Could you check a few things on this drawing? It's one solid part, dimensions in mm from its lowest x, y, z. Coordinates: 2 decimals unless noted, no trailing zeros. Write each loop counter-clockwise with the first axis right and the second up, starting at its lowest first coordinate (ties: lowest second). Pieces come first, ordered by that corner, then holes.
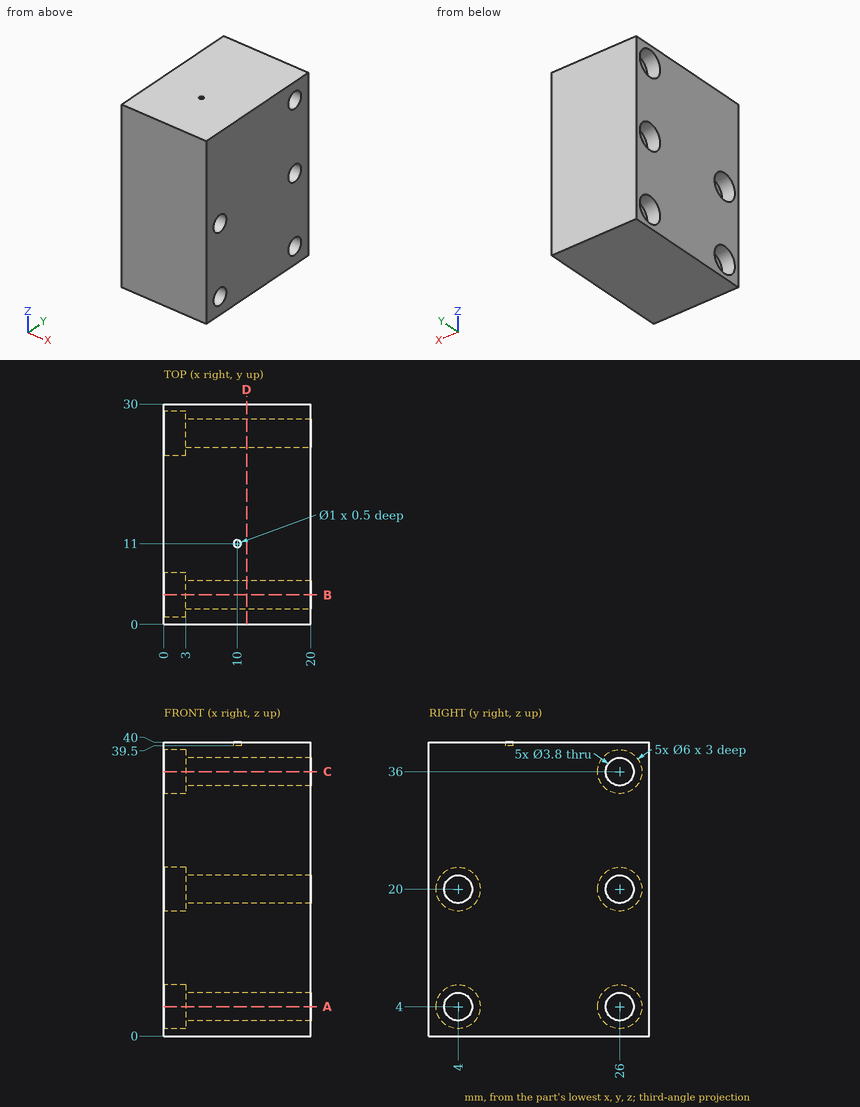
1) Imagine slicing it at C-C on z = 36. Please give me the cut outline in (x, y), then the cut area to 3 significant figures.
Values follow:
outline: (0, 0) - (20, 0) - (20, 24.1) - (3, 24.1) - (3, 23) - (0, 23) - close; (0, 29) - (3, 29) - (3, 27.9) - (20, 27.9) - (20, 30) - (0, 30) - close
area: 517 mm2
2) Imagine slicing it at A-A on z = 4. Please give me the cut outline in (x, y), then the cut area to 3 significant figures.
Values follow:
outline: (0, 0) - (20, 0) - (20, 2.1) - (3, 2.1) - (3, 1) - (0, 1) - close; (0, 7) - (3, 7) - (3, 5.9) - (20, 5.9) - (20, 24.1) - (3, 24.1) - (3, 23) - (0, 23) - close; (0, 29) - (3, 29) - (3, 27.9) - (20, 27.9) - (20, 30) - (0, 30) - close
area: 435 mm2
3) I need wall thicknesses on probe 1 along Z at (x, y) = (2.1, 4); probe 2 along Z at (x, y) = (1.5, 26); probe 3 along Z at (x, y) = (9.75, 26). Which ranges of each line are inside material? Lowest first, please.
Values follow:
probe 1: z = 0 to 1, 7 to 17, 23 to 40
probe 2: z = 0 to 1, 7 to 17, 23 to 33, 39 to 40
probe 3: z = 0 to 2.1, 5.9 to 18.1, 21.9 to 34.1, 37.9 to 40
4) Will these pins go through, and if not, where does the flat tip stop? pin 1 (3.5 mm diameter, centred on y = 4, z = 4, fed in from +X); pin 2 (5 mm diameter, centred on y = 26, z = 36, fed in from -X); pin 3 (0.5 mm diameter, centred on x = 10, y = 11, fed in from +Z).
Values follow:
pin 1: passes through
pin 2: stops at x = 3
pin 3: stops at z = 39.5
5) Imagine slicing it at D-D on x = 11.25. Please give me the cut outline in (y, z).
Values follow:
outline: (0, 0) - (30, 0) - (30, 40) - (0, 40) - close; hole circle Ø3.8 at (4, 4); hole circle Ø3.8 at (4, 20); hole circle Ø3.8 at (26, 4); hole circle Ø3.8 at (26, 20); hole circle Ø3.8 at (26, 36)
6) Imagine slicing it at B-B on y = 4. Please give me the cut outline in (x, z), then the cut area to 3 significant figures.
Values follow:
outline: (0, 0) - (20, 0) - (20, 2.1) - (3, 2.1) - (3, 1) - (0, 1) - close; (0, 7) - (3, 7) - (3, 5.9) - (20, 5.9) - (20, 18.1) - (3, 18.1) - (3, 17) - (0, 17) - close; (0, 23) - (3, 23) - (3, 21.9) - (20, 21.9) - (20, 40) - (0, 40) - close
area: 635 mm2
